Can you work these out from the model? Positions are in its coordinate system, mm. A direction names the side the tool comes from. Round coordinates to 2 decimals unless told otherwise and drop trailing zeros. Write each loop counter-clockwise with the first axis right and the second up, starting at its lowest first coordinate (ties: lowest second). Pieces come first, ordered by that corner, then holes. Notation, with made-up numbers: M 48,30.5 L 93,30.5 A25 ccw 93,43.5 Z; hole C 84.25,74 d11. An arc over 180 degrees is marked long. Answer as a JSON object with one key per item and string values. Group by question number.
1) On a 3-axis mill with a long thin cutter (end or side, diameter ignored), from which of +Z, -Z, +X, -X, +Y, -Y can I reach the whole of each face in a straight line? I mean faces 1 (the cylindrical face through (-12.6, 0.15, -77.15)), 2 (the cylindrical face through (28.092, 0.606, 3.116)), 3 (the flat face through (25.531, 4, 3)). Say none if no direction works.
2) Please list where these lines run through material, in increasing order: L1, parallel to X at y = 5.75, z = -5.5; L2, parallel to Z at x = -7, y = -9.5; L3, parallel to X at y = 5.5, z = 3. Write a range as [from, to].
3) If we mould it in two halves opening along X, with no side actions, what happens to faces 4 (the flat face through (34, 10.64, -80)), 5 (the flat face through (73.5, 0, -37)), 6 (the cylindrical face through (72.6, 0.15, -0.86)), 7 (the flat face through (78.5, 0, -38))? For each: +X half, -X half, draft (parallel to the pull), parting line (faces both ways), or undercut.
4) Suppose I cut it at B-B, the plane x = 30. Write out the boundary of the cut face in (y, z) (3 decimals), and give its area (3 significant figures).
5) I'm going to push a flat-ended pin straight in: pin 1 Ø7 at (x, z) = (20, 3) entering from +Y. Where does the tip first touch, or does it pass through?
6) Suppose I cut it at A-A, the plane z = -12. Write out the boundary of the cut face in (x, y).
7) Suppose I cut it at C-C, the plane y = 4.25. Write out the boundary of the cut face in (x, z).
from build123d import *

# Parameters (mm, degrees)
SKETCH1_W           = 60
SKETCH1_H           = 6.32
BOSS_EXTRUDE1_DEPTH = 10.64
SKETCH2_R           = 5
CUT_EXTRUDE1_DEPTH  = 64.974845056
SKETCH3_W           = 6.32
SKETCH3_H           = 21.28
BOSS_EXTRUDE2_DEPTH = 18.5
SKETCH4_W           = 6.32
SKETCH4_H           = 21.28
BOSS_EXTRUDE3_DEPTH = 18.5
SKETCH5_W           = 5
SKETCH5_H           = 21.28
BOSS_EXTRUDE6_DEPTH = 84.33
SKETCH6_W           = 5
SKETCH6_H           = 21.291954735
BOSS_EXTRUDE7_DEPTH = 84.33
SKETCH7_W           = 6.32
SKETCH7_H           = 21.291954735
BOSS_EXTRUDE8_DEPTH = 92
SKETCH9_R           = 5
CUT_EXTRUDE2_DEPTH  = 118.162904694
SKETCH10_R          = 2.22
CUT_EXTRUDE3_DEPTH  = 121.387443862
FILLET1_R           = 3
SKETCH13_R          = 2
CUT_EXTRUDE4_DEPTH  = 121.387443862
SKETCH14_W          = 12.9
SKETCH14_H          = 6.32
CUT_EXTRUDE5_DEPTH  = 12.7


with BuildPart() as part:
    # Sketch1 → Boss-Extrude1 (new, symmetric)
    with BuildSketch(Plane(origin=(0, 0, 0), x_dir=(1, 0, 0), z_dir=(0, 1, 0))):
        with Locations((30, -3.16)):
            Rectangle(SKETCH1_W, SKETCH1_H)
    extrude(amount=BOSS_EXTRUDE1_DEPTH, both=True)

    # Sketch2 → Cut-Extrude1 (cut, through all)
    with BuildSketch(Plane(origin=(0, 10.64, 0), x_dir=(1, 0, 0), z_dir=(0, 1, 0))):
        with Locations((7.21, 1.25)):
            Circle(SKETCH2_R)
        with Locations((52.79, 1.25)):
            Circle(SKETCH2_R)
    extrude(amount=-CUT_EXTRUDE1_DEPTH, mode=Mode.SUBTRACT)

    # Sketch3 → Boss-Extrude2 (add)
    with BuildSketch(Plane(origin=(60, 0, 0), x_dir=(0, 0, -1), z_dir=(1, 0, 0))):
        with Locations((-3.16, 0)):
            Rectangle(SKETCH3_W, SKETCH3_H)
    extrude(amount=BOSS_EXTRUDE2_DEPTH)

    # Sketch4 → Boss-Extrude3 (add)
    with BuildSketch(Plane.ZY):
        with Locations((3.16, 0)):
            Rectangle(SKETCH4_W, SKETCH4_H)
    extrude(amount=BOSS_EXTRUDE3_DEPTH)

    # Sketch5 → Boss-Extrude6 (add)
    with BuildSketch(Plane(origin=(0, 0, 0), x_dir=(-1, 0, 0), z_dir=(0, 0, -1))):
        with Locations((16, 0)):
            Rectangle(SKETCH5_W, SKETCH5_H)
    extrude(amount=BOSS_EXTRUDE6_DEPTH)

    # Sketch6 → Boss-Extrude7 (add)
    with BuildSketch(Plane(origin=(0, 0, 0), x_dir=(-1, 0, 0), z_dir=(0, 0, -1))):
        with Locations((-76, -0.005977367)):
            Rectangle(SKETCH6_W, SKETCH6_H)
    extrude(amount=BOSS_EXTRUDE7_DEPTH)

    # Sketch7 → Boss-Extrude8 (add, through all)
    with BuildSketch(Plane.ZY.offset(-73.5)):
        with Locations((-81.17, -0.005977367)):
            Rectangle(SKETCH7_W, SKETCH7_H)
    extrude(amount=BOSS_EXTRUDE8_DEPTH)

    # Sketch9 → Cut-Extrude2 (cut, through all)
    with BuildSketch(Plane(origin=(0, 10.64, 0), x_dir=(1, 0, 0), z_dir=(0, 1, 0))):
        with Locations((7.21, 76.76)):
            Circle(SKETCH9_R)
        with Locations((52.79, 76.76)):
            Circle(SKETCH9_R)
    extrude(amount=-CUT_EXTRUDE2_DEPTH, mode=Mode.SUBTRACT)

    # Sketch10 → Cut-Extrude3 (cut, through all)
    with BuildSketch(Plane(origin=(0, 0, -84.33), x_dir=(-1, 0, 0), z_dir=(0, 0, -1))):
        with Locations((-62.631229183, 0.005)):
            Circle(SKETCH10_R)
        with Locations((2.631229183, 0.005)):
            Circle(SKETCH10_R)
    extrude(amount=-CUT_EXTRUDE3_DEPTH, mode=Mode.SUBTRACT)

    # Fillet1
    fillet1_edges = [part.edges().sort_by_distance(p)[0] for p in [
        (78.5, 0, 6.32),
        (-18.5, 0, 6.32),
        (-13.5, 0, 0),
        (-18.5, -0.005977367, -84.33),
        (73.5, 0, 0),
        (78.5, -0.005977367, -84.33),
        (-13.5, 0, -78.01),
        (73.5, -0.005977367, -78.01),
    ]]
    fillet(fillet1_edges, radius=FILLET1_R)

    # Sketch13 → Cut-Extrude4 (cut, through all)
    with BuildSketch(Plane(origin=(0, 0, -84.33), x_dir=(-1, 0, 0), z_dir=(0, 0, -1))):
        with Locations((-30, 0.005)):
            Circle(SKETCH13_R)
    extrude(amount=-CUT_EXTRUDE4_DEPTH, mode=Mode.SUBTRACT)

    # Sketch14 → Cut-Extrude5 (cut, symmetric)
    with BuildSketch(Plane(origin=(0, 10.64, 0), x_dir=(1, 0, 0), z_dir=(0, 1, 0))):
        with Locations((19.080701294, -3.16)):
            Rectangle(SKETCH14_W, SKETCH14_H)
    extrude(amount=CUT_EXTRUDE5_DEPTH, both=True, mode=Mode.SUBTRACT)


solid = part.part
Results:
{
 "1": {"face 1": "+Y, -Y", "face 2": "+Z, -Z", "face 3": "+Z, +Y"},
 "2": {"L1": "[-18.5, -13.5], [73.5, 78.5]", "L2": "[-84.33, -78.01], [0, 6.32]", "L3": "[-18.5, 4.58], [9.84, 12.63], [25.53, 50.16], [55.42, 78.5]"},
 "3": {"face 4": "draft", "face 5": "undercut", "face 6": "undercut", "face 7": "+X half"},
 "4": {"outline": "M -10.652,-84.33 L -1.995,-84.33 L -1.995,-78.01 L -10.652,-78.01 Z; M -10.64,0 L -1.995,0 L -1.995,6.32 L -10.64,6.32 Z; M 2.005,-84.33 L 10.64,-84.33 L 10.64,-78.01 L 2.005,-78.01 Z; M 2.005,0 L 10.64,0 L 10.64,6.32 L 2.005,6.32 Z", "area": "218 mm^2"},
 "5": {"pin 1": "y = -2.06"},
 "6": {"outline": "M -18.5,-10.64 L -13.5,-10.64 L -13.5,10.64 L -18.5,10.64 Z; M 73.5,-10.65 L 78.5,-10.65 L 78.5,10.64 L 73.5,10.64 Z"},
 "7": {"outline": "M -18.5,-81.33 A3 ccw -15.5,-84.33 L 75.5,-84.33 A3 ccw 78.5,-81.33 L 78.5,3.32 A3 ccw 75.5,6.32 L 25.53,6.32 L 25.53,0 L 47.95,0 A5 cw 57.63,0 L 70.5,0 A3 cw 73.5,-3 L 73.5,-75.01 A3 cw 70.5,-78.01 L 57.63,-78.01 A5 cw 47.95,-78.01 L 12.05,-78.01 A5 cw 2.37,-78.01 L -10.5,-78.01 A3 cw -13.5,-75.01 L -13.5,-3 A3 cw -10.5,0 L 2.37,0 A5 cw 12.05,0 L 12.63,0 L 12.63,6.32 L -15.5,6.32 A3 ccw -18.5,3.32 Z"}
}
